Can you work these out from the model? Positions are in its coordinate system, mm. A direction names the side the tool comes from. Coordinates: 2 decimals unless noted, no trailing zeros. Loops run counter-clockwise (first coordinate to the right, second up) from the corner with the lowest first, then second, coordinate; pieces in that order, holes last. Notation, with made-up numbers: M 28,-9 L 80,-9 A13 ccw 80,13 Z; hole C 58.25,85 d5. An arc over 180 degrees is marked long. Answer as a JSON object with one key per item and string values. Group by question number.
Item 1: Which directions (+Z, -Z, +X, -X, +Y, -Y) give clear straight access to the entire face, cutting with the end or side of a thin tool? Please do faces 1 (the flat face through (-65, 31.5, 0)), 2 (the flat face through (50.152, -46, 0)), 3 (the flat face through (-56, 0, 5)).
Item 2: I'm going to push flat-ended pins straight in: pin 1 Ø1 at (x, z) = (52.5, -0.5) entering from +Y; pin 2 Ø2.5 at (y, z) = (-39.35, 0) entering from -X; pin 3 Ø1.5 at (x, z) = (-57.5, -2.5) entering from -Y; pin 4 Ø2.5 at (x, z) = (39.65, 0) entering from +Y. Where does each tip first touch, or does it pass through?
Item 3: Suppose I cut it at A-A (y = 24). Write out the boundary of the cut face in (x, z), then the cut area to 3 significant figures.
Item 4: If I drill on line 1 (X direction, y = 11.5, z = 0.5); line 2 (X direction, y = -47.5, z = 1), over which ranges is the centre line in solid material (lowest first)?
Item 5: We'd pull the mould along Y, two halves only. Please class faces 4 (the flat face through (53.15, 1, 0)), 5 (the flat face through (-58, -16, 0)), 6 (the cylindrical face through (54.99, -55.15, 0.07)): +Y half, -Y half, draft (parallel to the pull), parting line (faces both ways), or undercut.
```python
from build123d import *

# Parameters (mm, degrees)
BASE_DEPTH                     = 5
ARM_DEPTH                      = 5
CUT_EXTRUDE1_DEPTH             = 91.09217483320299
BOSS_EXTRUDE4_DEPTH            = 7
BOSS_EXTRUDE5_DEPTH            = 4
BOSS_EXTRUDE6_DEPTH            = 1
CLEARANCE_DEPTH                = 20
M2X0_4_TAPPED_HOLE1_AT_2_COUNT = 2
M2X0_4_TAPPED_HOLE1_AT_2_PITCH = 79
M2X0_4_TAPPED_HOLE2_AT_2_COUNT = 2
M2X0_4_TAPPED_HOLE2_AT_2_PITCH = 79
EXTENDER_DEPTH                 = 18.310000000000002
ANGLED_HORIZONTAL_DEPTH        = 30.405592
BOSS_EXTRUDE9_DEPTH            = 4
BOSS_EXTRUDE10_DEPTH           = 1
BOSS_EXTRUDE11_START           = -5
BOSS_EXTRUDE11_DEPTH           = 10
FILLET1_R                      = 1
FILLET2_R                      = 10
SPLIT1_START                   = -38.162950904
SPLIT1_DEPTH                   = 33.162950904


# Read off the part's stored shape, not the designer's step: Split1
with BuildPart() as part:
    # Sketch1 → base (new, symmetric)
    with BuildSketch(Plane.XY):
        Polygon((58.00000000000011, 58.00000000000005), (58.00000000000011, -58.00000000000005), (-58.00000000000008, -58.00000000000009), (-58.00000000000008, 58.00000000000009), align=None)
        Polygon((-41.5, 53.00000000000001), (41.5, 53.00000000000001), (41.5, 50.00188016), (50.00188015999998, 50.00188015999996), (50.00188015999998, 41.49999999999998), (52.999999999999986, 41.49999999999998), (52.999999999999986, -41.49999999999998), (50.00188015999996, -41.499999999999964), (50.00188015999999, -50.001880160000006), (41.499999999999964, -50.00188015999996), (41.49999999999998, -52.99999999999998), (-41.5, -53.00000000000001), (-41.5, -50.00188016), (-50.00188015999999, -50.001880160000006), (-50.00188015999996, -41.499999999999964), (-52.999999999999986, -41.49999999999998), (-52.999999999999986, 41.49999999999998), (-50.00188015999998, 41.49999999999998), (-50.00188015999998, 50.00188015999996), (-41.5, 50.00188016), align=None, mode=Mode.SUBTRACT)
    extrude(amount=BASE_DEPTH, both=True)

    # Sketch2 → arm (add, symmetric)
    with BuildSketch(Plane(origin=(0, 0, 0), x_dir=(0.7071067811865476, -0.7071067811865475, 0), z_dir=(0.7071067811865475, 0.7071067811865476, 0))):
        Polygon((70.9254691007821, 5), (82.02438661763962, 5), (82.02438661763962, 23.310000000000002), (5.0243866176396255, 23.30999999999999), (16.33438661763979, 12), (70.9254691007821, 12), align=None)
    extrude(amount=ARM_DEPTH, both=True)

    # Sketch3 → Cut-Extrude1 (cut, through all)
    with BuildSketch(Plane.XY):
        Polygon((54.81801948466061, -61.889087296526085), (61.88908729652609, -54.81801948466061), (58.00000000000011, -50.928932188134624), (58.0000000000001, -58.00000000000005), (50.92893218813458, -58.00000000000006), align=None)
    extrude(amount=-CUT_EXTRUDE1_DEPTH, mode=Mode.SUBTRACT)

    # Sketch5 → Boss-Extrude4 (add)
    with BuildSketch(Plane(origin=(0, 0, -5), x_dir=(-1, 0, 0), z_dir=(0, 0, -1))):
        Polygon((-50.15188015999995, -50.151880159999976), (-46.61634625406723, -53.68741406593269), (-43.080812348134494, -50.15188015999998), align=None)
        Polygon((-53.68741406593271, -46.61634625406722), (-50.15188015999995, -50.151880159999976), (-50.15188015999996, -43.08081234813448), align=None)
    extrude(amount=BOSS_EXTRUDE4_DEPTH)

    # Sketch9 → Boss-Extrude5 (add)
    with BuildSketch(Plane(origin=(10.01771845904714, -10.017718459047138, -14.167193308819991), x_dir=(0.8660254037844407, 0.2886751345948079, 0.40824829046386213), z_dir=(-0.4999999999999964, 0.4999999999999963, 0.7071067811865527))):
        Polygon((-9.25319791566329, -10.296687914526352), (12.79220976938526, 5.291769353593638), (-8.569750190631026, 35.50214284791941), (-30.61515787567957, 19.913685579799417), align=None)
        Polygon((-8.80889650236913, 34.10829599780206), (-29.221311025562215, 19.67453926806133), (-9.014051603925173, -8.902841064409014), (11.39836291926792, 5.530915665331709), align=None, mode=Mode.SUBTRACT)
    extrude(amount=BOSS_EXTRUDE5_DEPTH)

    # Sketch9<2> → Boss-Extrude6 (add)
    with BuildSketch(Plane(origin=(10.01771845904714, -10.017718459047138, -14.167193308819991), x_dir=(0.8660254037844407, 0.2886751345948079, 0.40824829046386213), z_dir=(-0.4999999999999964, 0.4999999999999963, 0.7071067811865527))):
        Polygon((-9.014051603925173, -8.902841064409014), (11.39836291926792, 5.530915665331709), (-8.80889650236913, 34.10829599780206), (-29.221311025562215, 19.67453926806133), align=None)
    extrude(amount=BOSS_EXTRUDE6_DEPTH)

    # Sketch7 → clearance (cut)
    with BuildSketch(Plane.XY.offset(15)):
        Polygon((-41.65, 53.150000000000006), (41.649999999999984, 53.150000000000006), (41.649999999999984, 50.15188016), (50.151880159999976, 50.15188016), (50.151880159999976, 41.64999999999998), (53.149999999999984, 41.64999999999998), (53.14999999999999, -41.64999999999996), (50.15188015999996, -41.64999999999996), (50.15188015999996, -50.15188015999998), (41.64999999999998, -50.15188015999998), (41.64999999999998, -53.14999999999998), (-41.65, -53.149999999999984), (-41.65, -50.15188016), (-50.15188015999999, -50.15188016), (-50.15188015999999, -41.64999999999998), (-53.149999999999984, -41.64999999999998), (-53.149999999999984, 41.64999999999998), (-50.151880159999976, 41.64999999999998), (-50.151880159999976, 50.15188015999996), (-41.65, 50.15188015999996), align=None)
    extrude(amount=-CLEARANCE_DEPTH, mode=Mode.SUBTRACT)

    # Sketch12 → M2x0.4 Tapped Hole1 (revolve, cut)
    with BuildSketch(Plane(origin=(-39.350000000000016, 0, 0), x_dir=(0, 0, -1), z_dir=(1, 0, 0))):
        Polygon((0, 0), (-1.421e-14, 58.00000000000009), (0.7999999999999855, 58.00000000000009), (0.7999999999999883, -1.46e-15), align=None)
    m2x0_4_tapped_hole1 = revolve(axis=Axis((-39.350000000000016, -6.349999999999991, 0), (0, 1, 0)), mode=Mode.SUBTRACT)

    # M2x0.4 Tapped Hole1 at 2: M2x0.4 Tapped Hole1 ×2
    with Locations(*[(i * M2X0_4_TAPPED_HOLE1_AT_2_PITCH, 0, 0) for i in range(1, M2X0_4_TAPPED_HOLE1_AT_2_COUNT)]):
        add(m2x0_4_tapped_hole1, mode=Mode.SUBTRACT)

    # Mirror1: M2x0.4 Tapped Hole1 across plane
    add(m2x0_4_tapped_hole1.mirror(Plane.ZX), mode=Mode.SUBTRACT)

    # Mirror1 copy 1 sketch → Mirror1 copy 1 (revolve, cut)
    with BuildSketch(Plane(origin=(39.649999999999984, 0, 0), x_dir=(0, 0, -1), z_dir=(1, 0, 0))):
        Polygon((0, 0), (-1.421e-14, -58.00000000000009), (0.7999999999999855, -58.00000000000009), (0.7999999999999883, 1.46e-15), align=None)
    revolve(axis=Axis((39.649999999999984, 6.349999999999991, 0), (0, 1, 0)), mode=Mode.SUBTRACT)

    # Sketch15 → M2x0.4 Tapped Hole2 (revolve, cut)
    with BuildSketch(Plane.ZX.offset(39.65)):
        Polygon((0, 0), (-1.421e-14, 58.00000000000011), (0.7999999999999923, 58.00000000000011), (0.7999999999999883, -1.46e-15), align=None)
    m2x0_4_tapped_hole2 = revolve(axis=Axis((-6.349999999999991, 39.65, 0), (1, 0, 0)), mode=Mode.SUBTRACT)

    # M2x0.4 Tapped Hole2 at 2: M2x0.4 Tapped Hole2 ×2
    with Locations(*[(0, -i * M2X0_4_TAPPED_HOLE2_AT_2_PITCH, 0) for i in range(1, M2X0_4_TAPPED_HOLE2_AT_2_COUNT)]):
        add(m2x0_4_tapped_hole2, mode=Mode.SUBTRACT)

    # Mirror2: M2x0.4 Tapped Hole2 across plane
    add(m2x0_4_tapped_hole2.mirror(Plane(origin=(0, 0, 0), x_dir=(0, 0, 1), z_dir=(1, 0, 0))), mode=Mode.SUBTRACT)

    # Mirror2 copy 1 sketch → Mirror2 copy 1 (revolve, cut)
    with BuildSketch(Plane.ZX.offset(-39.35)):
        Polygon((0, 0), (-1.421e-14, -58.00000000000011), (0.7999999999999923, -58.00000000000011), (0.7999999999999883, 1.46e-15), align=None)
    revolve(axis=Axis((6.349999999999991, -39.35, 0), (1, 0, 0)), mode=Mode.SUBTRACT)

    # Sketch16 → extender (add)
    with BuildSketch(Plane(origin=(0, 0, -5), x_dir=(-1, 0, 0), z_dir=(0, 0, -1))):
        Polygon((53.149999999999984, 21.649999999999977), (109.71854249492377, 78.21854249492374), (109.71854249492377, 68.21854249492375), (53.14999999999998, 11.649999999999949), align=None)
    extrude(amount=EXTENDER_DEPTH)

    # Sketch17 → angled horizontal (add)
    with BuildSketch(Plane(origin=(-15.749999999999996, -15.75, 0), x_dir=(0.7071067811865476, -0.7071067811865475, 0), z_dir=(0.7071067811865475, 0.7071067811865476, 0))):
        Polygon((-132.8915872327537, 23.310000000000006), (-132.8915872327537, 5), (-121.58158723275366, 5), (-121.58158723275366, 12), (-110.27158723275356, 23.310000000000006), align=None)
    extrude(amount=ANGLED_HORIZONTAL_DEPTH)

    # Sketch19 → Boss-Extrude9 (add)
    with BuildSketch(Plane(origin=(-47.228223086970885, 47.22822308697087, -66.79079361637689), x_dir=(0.8660254037844398, 0.2886751345948101, -0.4082482904638625), z_dir=(0.49999999999999806, -0.4999999999999979, 0.7071067811865506))):
        Polygon((-55.75778860387471, 55.47372790481981), (-34.39582864385848, 25.263354410494006), (-12.350420958809925, 40.85181167861396), (-33.71238091882616, 71.06218517293976), align=None)
        Polygon((-54.36394175375736, 55.234581593081714), (-33.95152723056426, 69.66833832282242), (-13.744267808927273, 41.09095799035208), (-34.15668233212039, 26.65720126061137), align=None, mode=Mode.SUBTRACT)
    extrude(amount=BOSS_EXTRUDE9_DEPTH)

    # Sketch19<2> → Boss-Extrude10 (add)
    with BuildSketch(Plane(origin=(-47.228223086970885, 47.22822308697087, -66.79079361637689), x_dir=(0.8660254037844398, 0.2886751345948101, -0.4082482904638625), z_dir=(0.49999999999999806, -0.4999999999999979, 0.7071067811865506))):
        Polygon((-34.15668233212039, 26.65720126061137), (-54.36394175375736, 55.234581593081714), (-33.95152723056426, 69.66833832282242), (-13.744267808927273, 41.09095799035208), align=None)
    extrude(amount=BOSS_EXTRUDE10_DEPTH)

    # Sketch21 → Boss-Extrude11 (add)
    with BuildSketch(Plane.XY.offset(BOSS_EXTRUDE11_START)):
        Polygon((-58.00000000000008, 16.500000000000064), (-58.00000000000008, 31.500000000000057), (-73.00000000000009, 31.500000000000057), align=None)
    extrude(amount=BOSS_EXTRUDE11_DEPTH)

    # Fillet1
    fillet1_edges = [part.edges().sort_by_distance(p)[0] for p in [
        (50.15188015999996, -50.151880159999976, -3.5),
        (-41.65, 50.15188015999996, 0),
        (41.649999999999984, 50.15188016, 0),
        (50.151880159999976, 50.15188016, 0),
        (50.151880159999976, 41.64999999999998, 0),
        (50.15188015999996, -41.64999999999996, 0),
        (41.64999999999998, -50.15188015999998, 0),
        (-41.65, -50.15188016, 0),
        (-50.15188015999999, -50.15188016, 0),
        (-50.15188015999999, -41.64999999999998, 0),
        (-50.151880159999976, 41.64999999999998, 0),
        (-50.151880159999976, 50.15188015999996, 0),
    ]]
    fillet(fillet1_edges, radius=FILLET1_R)

    # Fillet2
    fillet2_edges = [part.edges().sort_by_distance(p)[0] for p in [
        (58.0000000000001, -58.00000000000005, -9.155000000000001),
        (58.00000000000011, 58.00000000000005, 0),
        (-58.00000000000008, 58.00000000000009, 0),
        (-58.00000000000008, -58.00000000000009, 0),
    ]]
    fillet(fillet2_edges, radius=FILLET2_R)

    # Split1 outline → Split1 (cut)
    with BuildSketch(Plane.XY.offset(SPLIT1_START)):
        with BuildLine():
            Line((-53.15, 11.65), (-53.15, 34.058116908))
            Line((-53.15, 34.058116908), (31.059997068, -50.15188016))
            Line((31.059997068, -50.15188016), (43.080812348, -50.15188016))
            Line((43.080812348, -50.15188016), (50.588190451, -57.659258263))
            ThreePointArc((50.588190451, -57.659258263), (55.071067812, -55.071067812), (57.659258263, -50.588190451))
            Line((57.659258263, -50.588190451), (50.15188016, -43.080812348))
            Line((50.15188016, -43.080812348), (50.15188016, -31.059997068))
            Line((50.15188016, -31.059997068), (-53.15, 72.241883092))
            Line((-53.15, 72.241883092), (-53.15, 72.24432683))
            Line((-53.15, 72.24432683), (-76.424001385, 95.518328215))
            Line((-76.424001385, 95.518328215), (-80.2211648, 91.7211648))
            Line((-80.2211648, 91.7211648), (-88.218542495, 99.718542495))
            Line((-88.218542495, 99.718542495), (-109.718542495, 78.218542495))
            Line((-109.718542495, 78.218542495), (-109.718542495, 68.218542495))
            Line((-109.718542495, 68.218542495), (-53.15, 11.65))
        make_face()
    extrude(amount=SPLIT1_DEPTH, mode=Mode.SUBTRACT)


solid = part.part
```
From the geometry:
{
 "1": {"face 1": "+Z, -Z, -X, +Y", "face 2": "+Z, -Z", "face 3": "+Z, +X, -X, +Y, -Y"},
 "2": {"pin 1": "y = 57.17", "pin 2": "x = -58", "pin 3": "y = -52.84", "pin 4": "y = 58"},
 "3": {"outline": "M -65.5,-5 L -53.15,-5 L -53.15,5 L -65.5,5 Z; M 53.15,-5 L 58,-5 L 58,5 L 53.15,5 Z", "area": "172 mm2"},
 "4": {"line 1": "-58 to -53.15, 53.15 to 58", "line 2": "-58 to -50.15, 50.15 to 58"},
 "5": {"face 4": "undercut", "face 5": "draft", "face 6": "-Y half"}
}
